```python
from build123d import *

# Parameters (mm, degrees)
SKETCH_1_R          = 3
EXTRUDE_1_DEPTH     = 5
SKETCH_2_R          = 3
EXTRUDE_2_DEPTH     = 75
SKETCH_3_R          = 1.75
CUT_EXTRUDE_1_DEPTH = 81.280757346
CHAMFER_1_SIZE      = 1


with BuildPart() as part:
    # Эскиз1 → Бобышка-Вытянуть1 (new body)
    with BuildSketch(Plane.XY):
        Circle(SKETCH_1_R)
    extrude(amount=EXTRUDE_1_DEPTH)

    # Эскиз2 → Бобышка-Вытянуть2 (add)
    with BuildSketch(Plane.XY.offset(5)):
        Circle(SKETCH_2_R)
    extrude(amount=EXTRUDE_2_DEPTH)

    # Эскиз3 → Вырез-Вытянуть1 (cut, through all)
    with BuildSketch(Plane(origin=(3, 0, 0), x_dir=(0, 0, -1), z_dir=(1, 0, 0))):
        with Locations((-75, 0)):
            Circle(SKETCH_3_R)
        with Locations((-5, 0)):
            Circle(SKETCH_3_R)
    extrude(amount=-CUT_EXTRUDE_1_DEPTH, mode=Mode.SUBTRACT)

    # Фаска1
    chamfer_1_edges = [part.edges().sort_by_distance(p)[0] for p in [
        (-3, 0, 0),
        (-3, 0, 80),
    ]]
    chamfer(chamfer_1_edges, length=CHAMFER_1_SIZE)


solid = part.part
```
Design review of the part built by this model. Coordinates are the model's own, in mm. Give positions to 0.01 mm unless a question says otherwise; leave off trailing zeros. Write each loop counter-clockwise with the first axis right and the second up, starting at its lowest first coordinate (ties: lowest second). Pieces come first, ordered by that corner, then holes.
(1) Wall thickness on line 1 along Z through (x, y) = (1.25, 0); line 2 along Z through (x, y) = (0.5, 1); line 3 along Y through (x, z) = (-1.25, 5): over which ranges is each line inside the solid? List them lowest first.
Checked values:
line 1: z = 0 to 3.25, 6.75 to 73.25, 76.75 to 80
line 2: z = 0 to 3.56, 6.44 to 73.56, 76.44 to 80
line 3: y = -2.73 to -1.75, 1.75 to 2.73
(2) Add section D-D (z = 75). Give the boundary of the cut face in (x, y), and give its area (4 significant figures).
Checked values:
outline: (-2.44, -1.75) arc R3 ccw to (2.44, -1.75) - close; (-2.44, 1.75) - (2.44, 1.75) arc R3 ccw to start
area: 8.535 mm2
(3) Clearance check with flat-ended pins moving along their axes: pin 1 Ø1.5 at (y, z) = (-1.5, 67.5) entering from -X; pin 2 Ø1.5 at (y, z) = (-1, 46.5) entering from +X; pin 3 Ø1 at (x, z) = (1, 31.5) entering from -Y. State where each tip first meets the part, or that it passes through.
Checked values:
pin 1: stops at x = -2.9
pin 2: stops at x = 2.99
pin 3: stops at y = -2.96
(4) Mouldability with a two-part tool opening along Z and no side actions: class faces 1 (the face through (0, 0, 80)), 2 (the face through (0, 0, 0)), 3 (the face through (0.04, 0.08, 6.75)) as +Z half, -Z half, draft (parallel to the pull), parting line (faces both ways), or undercut.
Checked values:
face 1: +Z half
face 2: -Z half
face 3: undercut
(5) Add section C-C (z = 19.5). Give the boundary of the cut face in (x, y), and give its area (3 significant figures).
Checked values:
outline: circle Ø6 at (0, 0)
area: 28.3 mm2
(6) Add section A-A (y = 0). Give the boundary of the cut face in (x, z).
Checked values:
outline: (-3, 1) - (-2, 0) - (2, 0) - (3, 1) - (3, 3.25) - (-3, 3.25) - close; (-3, 6.75) - (3, 6.75) - (3, 73.25) - (-3, 73.25) - close; (-3, 76.75) - (3, 76.75) - (3, 79) - (2, 80) - (-2, 80) - (-3, 79) - close
(7) Add section B-B (x = 0). Give the boundary of the cut face in (y, z), and give its area (3 significant figures).
Checked values:
outline: (-3, 1) - (-2, 0) - (2, 0) - (3, 1) - (3, 79) - (2, 80) - (-2, 80) - (-3, 79) - close; hole circle Ø3.5 at (0, 5); hole circle Ø3.5 at (0, 75)
area: 459 mm2
